from build123d import *

# Parameters (mm, degrees)
BOSS_EXTRUDE1_DEPTH = 38.1
SKETCH4_R           = 17.78
SKETCH4_R_2         = 13.97
BOSS_EXTRUDE3_DEPTH = 12.7
SKETCH5_R           = 3.175
CUT_EXTRUDE2_DEPTH  = 12.7


with BuildPart() as part:
    # Sketch1 → Boss-Extrude1 (new body)
    with BuildSketch(Plane.XY):
        Polygon((-29.021915902, 16.755810958), (-29.021915902, 23.105810958), (29.021915902, 23.105810958), (29.021915902, 16.755810958), (0, 0), align=None)
    extrude(amount=BOSS_EXTRUDE1_DEPTH)

    # Sketch4 → Boss-Extrude3 (add)
    with BuildSketch(Plane(origin=(0, 0, 0), x_dir=(0.8660254037844379, -0.5000000000000012, 0), z_dir=(-0.5000000000000012, -0.8660254037844379, 0))):
        with Locations(Location((-16.755810958, 19.05, 0), (0, 0, 160.458003801))):
            Circle(SKETCH4_R)
        with Locations((-16.755810958, 19.05)):
            Circle(SKETCH4_R_2, mode=Mode.SUBTRACT)
    boss_extrude3 = extrude(amount=BOSS_EXTRUDE3_DEPTH)

    # Mirror2: Boss-Extrude3 across plane
    add(boss_extrude3.mirror(Plane.ZY))

    # Sketch5 → Cut-Extrude2 (cut)
    with BuildSketch(Plane(origin=(0, 23.105810958, 0), x_dir=(1, 0, 0), z_dir=(0, 1, 0))):
        with Locations(Location((-22.671915902, -19.05, 0), (0, 0, 270))):
            Circle(SKETCH5_R)
        with Locations(Location((15.428084098, -19.05, 0), (0, 0, 270))):
            Circle(SKETCH5_R)
    extrude(amount=-CUT_EXTRUDE2_DEPTH, mode=Mode.SUBTRACT)


solid = part.part
Design review of the part built by this model. Coordinates are the model's own, in mm. A direction names the side the tool comes from. Round coordinates to 2 decimals unless told otherwise and drop trailing zeros. Loops run counter-clockwise (first coordinate to the right, second up) from the corner with the lowest first, then second, coordinate; pieces in that order, holes last. Notation, with made-up numbers: (-5, 88) - (48, 88) arc R28 ccw to (48, 112) - close; hole circle Ø8 at (20.25, 50.5). An arc over 180 degrees is marked (long way). One line per question, with ' | ' between items.
1. We need section C-C, the plane y = 9.5. State how many separate pieces and enclosed holes the cut face has, and give its area (3 significant figures).
Results are:
separate pieces: 1 | enclosed holes: 2 | area: 1,650 mm²
2. We need section B-B, the plane z = 8. State the section outline as (x, y) points.
Results are:
outline: (-32.92, 4.34) - (-28.26, 1.65) - (-21.91, 12.65) - (-7.11, 4.1) - (-13.46, -6.89) - (-8.8, -9.59) - (-2.45, 1.41) - (0, 0) - (2.45, 1.41) - (8.8, -9.59) - (13.46, -6.89) - (7.11, 4.1) - (21.91, 12.65) - (28.26, 1.65) - (32.92, 4.34) - (26.57, 15.34) - (29.02, 16.76) - (29.02, 23.11) - (-29.02, 23.11) - (-29.02, 16.76) - (-26.57, 15.34) - close
3. For L1, parallel to X at y = 19.5, z = 19.05; L2, parallel to X at y = 5.5, z = 30; L3, parallel to X at y = 14, z = 19, list the stretches that pass through material, from the lowest coordinate up. Write a range as [from, to].
Results are:
L1: x = [-29.02, -25.85], [-19.5, 12.25], [18.6, 29.02] | L2: x = [-32.35, -26.19], [-9.53, 9.53], [26.19, 32.35] | L3: x = [-31.8, -27.4], [-19.5, 12.25], [18.6, 24.25], [27.4, 31.8]
4. Draft analysis for pull direction X (two halves, no side actions). For faces 6 (the face through (20.859, 4.813, 1.663)), 7 (the face through (-20.859, 4.813, 1.663)), 8 (the face through (0, 14, 0)), 9 (the face through (23.833, -0.905, 32.758)), state which applies: released by +X, released by -X, zero draft, split by the parting line, or undercut.
Results are:
face 6: undercut | face 7: undercut | face 8: zero draft | face 9: released by +X
5. Clearance check with flat-ended pins moving along their axes: P1, Ø3, axis at x = 25.5, y = 4.5, coming from the +Z side; P2, Ø8, axis at y = -1, z = 23.5, coming from the +X side; P3, Ø12, axis at y = 16.5, z = 22, coming from the +X side. State where each tip first meets the part, or that it passes through.
Results are:
P1: stops at z = 35.76 | P2: stops at x = 7.81 | P3: stops at x = 33.65
6. We need section D-D, the plane z = 23. State the section outline as (x, y) points.
Results are:
outline: (-35.87, 6.05) - (-32.47, 4.08) - (-26.12, 15.08) - (-2.91, 1.68) - (-9.26, -9.32) - (-5.85, -11.29) - (0, -1.16) - (5.85, -11.29) - (9.26, -9.32) - (2.91, 1.68) - (26.12, 15.08) - (32.47, 4.08) - (35.87, 6.05) - (29.52, 17.05) - (29.02, 16.76) - (29.02, 23.11) - (-29.02, 23.11) - (-29.02, 16.76) - (-29.52, 17.05) - close
7. For faces 1 (the face through (-14.443, 8.339, 0.697)), 2 (the face through (14.68, 8.476, 18.854)), 3 (the face through (14.58, 8.42, 37.34)), 4 (the face through (15.57, 16.84, 15.88)), 5 (the face through (0, 14, 38.1)), list the 3-axis set-ups (+Z, -Z, +X, -X, +Y, -Y) from which the entire face can be reached by the end or side of a thin tool; tool diameter is ignored.
Results are:
face 1: -Z | face 2: none | face 3: +Z | face 4: +Y | face 5: +Z, +X, -X, +Y, -Y
8. We need section A-A, the plane z = 19.05. State the section outline as (x, y) points, and give its area (3 significant figures).
Results are:
outline: (-36.26, 6.27) - (-32.96, 4.36) - (-26.61, 15.36) - (-25.85, 14.92) - (-25.85, 23.11) - (-29.02, 23.11) - (-29.02, 16.76) - (-29.91, 17.27) - close; (-19.5, 11.26) - (-2.41, 1.39) - (-8.76, -9.61) - (-5.46, -11.51) - (0, -2.05) - (5.46, -11.51) - (8.76, -9.61) - (2.41, 1.39) - (18.02, 10.41) - (12.25, 10.41) - (12.25, 23.11) - (-19.5, 23.11) - close; (18.6, 10.74) - (26.61, 15.36) - (32.96, 4.36) - (36.26, 6.27) - (29.91, 17.27) - (29.02, 16.76) - (29.02, 23.11) - (18.6, 23.11) - close | area: 902 mm²
